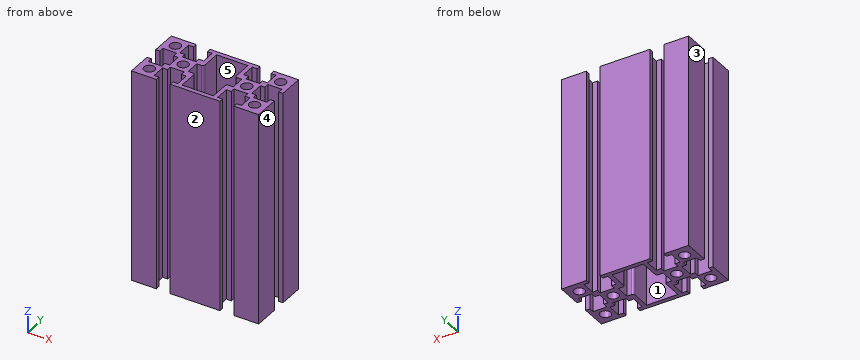
```python
from build123d import *

# Parameters (mm, degrees)
SKETCH_1_R      = 2.5
EXTRUDE_1_DEPTH = 100


with BuildPart() as part:
    # 草图1 → 凸台-拉伸1 (new body)
    with BuildSketch(Plane.XY):
        Polygon((-15, 15), (-3.25, 15), (-3.25, 13), (-5.6, 13), (-5.6, 6.5), (-3.25, 6.5), (-3.25, 4.4), (3.25, 4.4), (3.25, 6.5), (5.6, 6.5), (5.6, 13), (3.25, 13), (3.25, 15), (26.75, 15), (26.75, 13), (24.4, 13), (24.4, 6.5), (26.75, 6.5), (26.75, 4.4), (33.25, 4.4), (33.25, 6.5), (35.6, 6.5), (35.6, 13), (33.25, 13), (33.25, 15), (45, 15), (45, 3.25), (43, 3.25), (43, 5.6), (36.5, 5.6), (36.5, 3.25), (34.4, 3.25), (34.4, -3.25), (36.5, -3.25), (36.5, -5.6), (43, -5.6), (43, -3.25), (45, -3.25), (45, -15), (33.25, -15), (33.25, -13), (35.6, -13), (35.6, -6.5), (33.25, -6.5), (33.25, -4.4), (26.75, -4.4), (26.75, -6.5), (24.4, -6.5), (24.4, -13), (26.75, -13), (26.75, -15), (3.25, -15), (3.25, -13), (5.6, -13), (5.6, -6.5), (3.25, -6.5), (3.25, -4.4), (-3.25, -4.4), (-3.25, -6.5), (-5.6, -6.5), (-5.6, -13), (-3.25, -13), (-3.25, -15), (-15, -15), (-15, -3.25), (-13, -3.25), (-13, -5.6), (-6.5, -5.6), (-6.5, -3.25), (-4.4, -3.25), (-4.4, 3.25), (-6.5, 3.25), (-6.5, 5.6), (-13, 5.6), (-13, 3.25), (-15, 3.25), align=None)
        Circle(SKETCH_1_R, mode=Mode.SUBTRACT)
        with Locations((30, 0)):
            Circle(SKETCH_1_R, mode=Mode.SUBTRACT)
        with Locations((39.8, 9.8)):
            Circle(SKETCH_1_R, mode=Mode.SUBTRACT)
        with Locations((39.8, -9.8)):
            Circle(SKETCH_1_R, mode=Mode.SUBTRACT)
        with Locations((-9.8, 9.8)):
            Circle(SKETCH_1_R, mode=Mode.SUBTRACT)
        with Locations((-9.8, -9.8)):
            Circle(SKETCH_1_R, mode=Mode.SUBTRACT)
        with BuildLine():
            Line((7.6, 13), (7.6, 4.25))
            ThreePointArc((7.6, 4.25), (7.307106781, 3.542893219), (6.6, 3.25))
            Line((6.6, 3.25), (4.4, 3.25))
            Line((4.4, 3.25), (4.4, -3.25))
            Line((4.4, -3.25), (6.6, -3.25))
            ThreePointArc((6.6, -3.25), (7.307106781, -3.542893219), (7.6, -4.25))
            Line((7.6, -4.25), (7.6, -13))
            Line((7.6, -13), (22.4, -13))
            Line((22.4, -13), (22.4, -4.25))
            ThreePointArc((22.4, -4.25), (22.692893219, -3.542893219), (23.4, -3.25))
            Line((23.4, -3.25), (25.6, -3.25))
            Line((25.6, -3.25), (25.6, 3.25))
            Line((25.6, 3.25), (23.4, 3.25))
            ThreePointArc((23.4, 3.25), (22.692893219, 3.542893219), (22.4, 4.25))
            Line((22.4, 4.25), (22.4, 13))
            Line((22.4, 13), (7.6, 13))
        make_face(mode=Mode.SUBTRACT)
    extrude(amount=EXTRUDE_1_DEPTH)


solid = part.part
```
Here's how the part is built. I have some questions about the finished solid (model axes, mm). Face numbers are marked on the shaded views. A direction names the side the tool comes from. Round coordinates to 2 decimals unless told otherwise and drop trailing zeros. Order: outer loops, then holes, each group sorted by start corner. A loop starts at its lowest first (then second) coordinate and runs counter-clockwise, first axis right, second up. Notation, with made-up numbers: (87.5, 13.25) -> (118.5, 13.25) arc R11 cw to (118.5, 25.25) -> close; hole circle Ø6 at (24.25, -32). An arc over 180 degrees is marked (long way). Use a Markdown table: item, result. Add a question column.
(1) If we mould it in two halves opening along X, with no side actions, what happens to the marked faces 1, 2 and 3? For each: released by +X, released by -X, zero draft, split by the parting line, or undercut.
(2) Suppose I cut it at A-A, the plane y = 0. Please give me the cut outline in (x, z), and give its area (3 significant figures).
(3) Suppose I cut it at C-C, the plane y = 9.8. Please give me the cut outline in (x, z), and give its area (3 significant figures).
(4) For the marked faces 4 and 5, which set-ups out of +Z, -Z, +X, -X, +Y, -Y let a thin tool reach every point of the face, with its end or its side?
(5) Suppose I cut it at B-B, the plane x = 0. Please give me the cut outline in (y, z).
(6) I need wall thicknesses on line 1 along Y through (x, z) = (-5, 84); line 2 along Y through (x, z) = (-9.8, 22); line 3 along X through (y, z) = (6.25, 54.5). Which ranges of each line are inside material? Lowest first, please.
(7) Suppose I cut it at D-D, the plane x = 13. Please give me the cut outline in (y, z), and give its area (3 significant figures).
Verdict:
| question | item | result |
|---|---|---|
| 1 | face 1 | undercut |
| 1 | face 2 | zero draft |
| 1 | face 3 | released by -X |
| 2 | outline | (-4.4, 0) -> (-2.5, 0) -> (-2.5, 100) -> (-4.4, 100) -> close; (2.5, 0) -> (4.4, 0) -> (4.4, 100) -> (2.5, 100) -> close; (25.6, 0) -> (27.5, 0) -> (27.5, 100) -> (25.6, 100) -> close; (32.5, 0) -> (34.4, 0) -> (34.4, 100) -> (32.5, 100) -> close |
| 2 | area | 760 mm2 |
| 3 | outline | (-15, 0) -> (-12.3, 0) -> (-12.3, 100) -> (-15, 100) -> close; (-7.3, 0) -> (-5.6, 0) -> (-5.6, 100) -> (-7.3, 100) -> close; (5.6, 0) -> (7.6, 0) -> (7.6, 100) -> (5.6, 100) -> close; (22.4, 0) -> (24.4, 0) -> (24.4, 100) -> (22.4, 100) -> close; (35.6, 0) -> (37.3, 0) -> (37.3, 100) -> (35.6, 100) -> close; (42.3, 0) -> (45, 0) -> (45, 100) -> (42.3, 100) -> close |
| 3 | area | 1,280 mm2 |
| 4 | face 4 | +Z, -Z, +X, +Y, -Y |
| 4 | face 5 | +Z, -Z |
| 5 | outline | (-4.4, 0) -> (-2.5, 0) -> (-2.5, 100) -> (-4.4, 100) -> close; (2.5, 0) -> (4.4, 0) -> (4.4, 100) -> (2.5, 100) -> close |
| 6 | line 1 | -15 to -13, -6.5 to -3.25, 3.25 to 6.5, 13 to 15 |
| 6 | line 2 | -15 to -12.3, -7.3 to -5.6, 5.6 to 7.3, 12.3 to 15 |
| 6 | line 3 | -15 to -3.25, 3.25 to 7.6, 22.4 to 26.75, 33.25 to 45 |
| 7 | outline | (-15, 0) -> (-13, 0) -> (-13, 100) -> (-15, 100) -> close; (13, 0) -> (15, 0) -> (15, 100) -> (13, 100) -> close |
| 7 | area | 400 mm2 |
